CAD build for the part. Positions are in the model's coordinates, mm. Coordinates: 2 decimals unless noted, no trailing zeros. Loops run counter-clockwise (first coordinate to the right, second up) from the corner with the lowest first, then second, coordinate; pieces in that order, holes last. Notation, with made-up numbers: (7, 37) -> (21, 37) arc R26 cw to (21, 55) -> close; hole circle Ø8 at (76.25, 75.25). An arc over 180 degrees is marked (long way). Write item = value, one per line. Start each with the question number.
(1) Band-saw the part on A-A (z = -25). Write the cut outline in (x, y), and give its area (4 significant figures).
(2) Drill centre lines: line 1 (Z direction, x = -30, y = 5.25); line 2 (X direction, y = 6.25, z = -13); line 3 (X direction, y = 6.25, z = -35). Where is each one in solid material? Low to high. Write a range as from..to.
(3) Band-saw the part on C-C (y = 7.25). Write the cut outline in (x, z), and give its area (3 significant figures).
(4) Band-saw the part on B-B (x = -250). Write the cut outline in (y, z), and give its area (3 significant figures).
(5) Pull direction X, two halves, no side cores. Call faces 1 (the face through (0, 4, -25)), 2 (the face through (-136, 9, -25)), 3 (the face through (-263.856, 4.437, -19.255)): +X half, -X half, draft (parallel to the pull), parting line (faces both ways), or undercut.
(6) Band-saw the part on D-D (z = -36). Write the cut outline in (x, y), and give its area (3 significant figures).
(7) Flat gauge pin, fed straight in: P1, Ø3, axis at x = -190.5, z = -25, coming from the -Y side. Where does the tip first touch, or does it go through?
Autodesk Inventor part; units mm, degrees
ref_plane "YZ Plane" through (0, 0, 0) normal (1, 0, 0) x (0, 1, 0)
ref_plane "XZ Plane" through (0, 0, 0) normal (0, 1, 0) x (-1, 0, 0)
ref_plane "XY Plane" through (0, 0, 0) normal (0, 0, 1) x (1, 0, 0)
sketch "Skizze1" plane through (0, 0, 0) normal (0, 1, 0) x (-1, 0, 0)
  line L0 (0, 0) -> (275, 0)
  line L1 (275, 0) -> (275, -50)
  line L2 (275, -50) -> (0, -50)
  line L3 (0, -50) -> (0, 0)
  line L4 (275, 0) -> (275, -25)
  line L5 (275, -25) -> (250, -25)
  circle A0 centre (250, -25) radius 15
  dimension "d0" = 275
  dimension "d1" = 50
  dimension "d2" = 25
  dimension "d3" = 30
extrude "Extrusion1" add sketch "Skizze1" along normal blind 9
sketch "Skizze2" plane through (0, 9, 0) normal (0, 1, 0) x (1, 0, 0)
  line L0 (0, 0) -> (0, 50)
  line L1 (0, 50) -> (-30, 50)
  line L2 (-30, 50) -> (-30, 35)
  line L3 (0, 0) -> (-55, 0)
  line L4 (-275, 0) -> (0, 0)
  line L5 (-55, 0) -> (-70, 0)
  line L6 (-70, 0) -> (-55, 0)
  line L7 (-55, 0) -> (-55, 15)
  dimension "d6" = 30
  dimension "d7" = 15
  dimension "d8" = 55
  dimension "d9" = 15
  dimension "d10" = 15
hole "Bohrung1" at (-55, 9, -15) at (-30, 9, -35) direction (0, -1, 0) diameter 10 depth 10 tip angle 118
properties part number "Lagerstuetze_kurz" material "Holz (Birke)"
Findings below:
q1.outline = (-275, 0) -> (-265, 0) -> (-265, 9) -> (-275, 9) -> close; (-235, 0) -> (0, 0) -> (0, 9) -> (-235, 9) -> close
q1.area = 2,205 mm²
q2.line_1 = -50..-40, -30..0
q2.line_2 = -275..-259, -241..-59.58, -50.42..0
q2.line_3 = -275..-261.18, -238.82..-35, -25..0
q3.outline = (-275, -50) -> (0, -50) -> (0, 0) -> (-275, 0) -> close; hole circle Ø30 at (-250, -25); hole circle Ø10 at (-55, -15); hole circle Ø10 at (-30, -35)
q3.area = 12,900 mm²
q4.outline = (0, -50) -> (9, -50) -> (9, -40) -> (0, -40) -> close; (0, -10) -> (9, -10) -> (9, 0) -> (0, 0) -> close
q4.area = 180 mm²
q5.face_1 = +X half
q5.face_2 = draft
q5.face_3 = undercut
q6.outline = (-275, 0) -> (-260.2, 0) -> (-260.2, 9) -> (-275, 9) -> close; (-239.8, 0) -> (-34.9, 0) -> (-34.9, 9) -> (-239.8, 9) -> close; (-25.1, 0) -> (0, 0) -> (0, 9) -> (-25.1, 9) -> close
q6.area = 2,200 mm²
q7.P1 = 0
